Autodesk Inventor part; units mm, degrees
ref_plane "YZ Plane" through (0, 0, 0) normal (1, 0, 0) x (0, 1, 0)
ref_plane "XZ Plane" through (0, 0, 0) normal (0, 1, 0) x (-1, 0, 0)
ref_plane "XY Plane" through (0, 0, 0) normal (0, 0, 1) x (1, 0, 0)
sketch "Sketch1" plane through (0, 0, 0) normal (0, 0, 1) x (1, 0, 0)
  line L0 (0, 0) -> (20, 0)
  line L1 (20, 0) -> (20, -10)
  line L2 (20, -10) -> (0, -10)
  line L3 (0, -10) -> (0, 0)
  dimension "d0" = 20
  dimension "d1" = 10
extrude "Extrusion1" add sketch "Sketch1" along normal blind 6
sketch "Sketch2" plane through (0, 0, 0) normal (0, 1, 0) x (1, 0, 0)
  line L0 (20, 0) -> (20, -6)
  line L1 (20, 0) -> (10, 0)
  line L2 (10, 0) -> (10, -6)
  line L3 (10, -6) -> (20, -6)
  line L4 (20, -6) -> (20, 0)
  point P0 (0, 0)
  dimension "d4" = 10
extrude "Extrusion2" add sketch "Sketch2" along normal blind 1
chamfer "Chamfer2" distance 1 angle 45 1 edges at (10, 1, 3)
sketch "Sketch3" plane through (0, -10, 0) normal (0, -1, 0) x (1, 0, 0)
  line L0 (0, 6) -> (3, 6) construction
  line L1 (3, 6) -> (3, 0) construction
  line L2 (3, 0) -> (0, 0) construction
  line L3 (0, 0) -> (0, 6) construction
  line L4 (3, 6) -> (7, 6)
  line L5 (7, 6) -> (7, 0)
  line L6 (7, 0) -> (3, 0)
  line L7 (3, 0) -> (3, 6)
  line L8 (7, 6) -> (13, 6) construction
  line L9 (13, 6) -> (13, 0) construction
  line L10 (13, 0) -> (7, 0) construction
  line L11 (7, 0) -> (7, 6) construction
  line L12 (13, 6) -> (17, 6)
  line L13 (17, 6) -> (17, 0)
  line L14 (17, 0) -> (13, 0)
  line L15 (13, 0) -> (13, 6)
  dimension "d13" = 3
  dimension "d14" = 4
  dimension "d15" = 6
  dimension "d16" = 4
extrude "Extrusion3" add sketch "Sketch3" along normal blind 1
chamfer "Chamfer3" distance 1 angle 45 4 edges at (3, -11, 3) (7, -11, 3) (13, -11, 3) (17, -11, 3)
sketch "Sketch4" plane through (0, -10, 0) normal (0, -1, 0) x (1, 0, 0)
  line L0 (0, 6) -> (2.9323, 6) construction
  line L1 (0, 5) -> (2.9323, 5) construction
  line L2 (0, 0) -> (2.9323, 0) construction
  line L3 (2.9323, 1) -> (1, 1) construction
  line L4 (1, 1) -> (1, 5) construction
  line L5 (1, 5) -> (2.9323, 5) construction
  line L6 (2, 5) -> (2, 1) construction
  line L7 (1, 5) -> (2, 5)
  line L8 (2, 5) -> (2, 1)
  line L9 (2, 1) -> (1, 1)
  line L10 (1, 1) -> (1, 5)
  dimension "d22" = 1
  dimension "d23" = 1
  dimension "d24" = 1
extrude "Extrusion4" cut sketch "Sketch4" against normal blind 1
sketch "Sketch5" plane through (7, -10, 0) normal (0, -1, 0) x (1, 0, 0)
  line L0 (0, 0.2008) -> (0, 5.4827) construction
  line L1 (3, 0.2008) -> (3, 5.4827) construction
  line L2 (4, 0.2008) -> (4, 5.4827) construction
  line L3 (6, 0) -> (0.2208, 0) construction
  line L4 (6, 1) -> (0.2208, 1) construction
  line L5 (6, 6) -> (0.5976, 6) construction
  line L6 (6, 5) -> (0.5976, 5) construction
  line L7 (4, 1) -> (3, 1)
  line L8 (3, 1) -> (3, 5)
  line L9 (3, 5) -> (4, 5)
  line L10 (4, 5) -> (4, 1)
  point P0 (-7, 0)
  dimension "d27" = 3
  dimension "d28" = 1
  dimension "d29" = 1
  dimension "d30" = 1
extrude "Extrusion5" cut sketch "Sketch5" against normal blind 1
sketch "Sketch6" plane through (20, -10, 0) normal (0, -1, 0) x (1, 0, 0)
  line L0 (0, 0) -> (0, 5.7185) construction
  line L1 (-1, 0) -> (-1, 5.7185) construction
  line L2 (-2, 0) -> (-2, 5.7185) construction
  line L3 (-0.3844, 0) -> (-2.7356, 0) construction
  line L4 (-0.3844, 1) -> (-2.7356, 1) construction
  line L5 (-0.4485, 6) -> (-2.495, 6) construction
  line L6 (-0.4485, 5) -> (-2.495, 5) construction
  line L7 (-1, 1) -> (-2, 1)
  line L8 (-2, 1) -> (-2, 5)
  line L9 (-2, 5) -> (-1, 5)
  line L10 (-1, 5) -> (-1, 1)
  point P0 (-20, 0)
  dimension "d33" = 1
  dimension "d34" = 1
  dimension "d35" = 1
  dimension "d36" = 1
extrude "Extrusion6" cut sketch "Sketch6" against normal blind 1
sketch "Sketch7" plane through (0, 1, 0) normal (0, 1, 0) x (1, 0, 0)
  line L0 (11, -5.3093) -> (11, -0.576) construction
  line L1 (12.5, -5.3093) -> (12.5, -0.576) construction
  line L2 (14.5, -5.3093) -> (14.5, -0.576) construction
  line L3 (15, 0) -> (12.0712, 0) construction
  line L4 (15, -2) -> (12.0712, -2) construction
  line L5 (15, -4) -> (12.0712, -4) construction
  line L6 (14.5, -4) -> (12.5, -4)
  line L7 (12.5, -4) -> (12.5, -2)
  line L8 (12.5, -2) -> (14.5, -2)
  line L9 (14.5, -2) -> (14.5, -4)
  point P0 (0, 0)
  dimension "d39" = 1.5
  dimension "d40" = 2
  dimension "d41" = 2
  dimension "d42" = 2
extrude "Extrusion7" add sketch "Sketch7" along normal blind 1.5
sketch "Sketch8" plane through (0, 1, 0) normal (0, 1, 0) x (1, 0, 0)
  line L0 (14.5, -5.3842) -> (14.5, -1) construction
  line L1 (17.5, -5.3842) -> (17.5, -1) construction
  line L2 (18.8144, -6) -> (15.3684, -6) construction
  line L3 (18.8144, -5) -> (14.5, -5) construction
  line L4 (18.8144, -1) -> (14.5, -1) construction
  line L5 (17.5, -5) -> (18.5, -5)
  line L6 (18.5, -5) -> (18.5, -1)
  line L7 (18.5, -1) -> (17.5, -1)
  line L8 (17.5, -1) -> (17.5, -5)
  point P0 (0, 0)
  dimension "d45" = 3
  dimension "d47" = 1
  dimension "d48" = 4
  dimension "d49" = 1
extrude "Extrusion8" cut sketch "Sketch8" against normal blind 1
sketch "Sketch9" plane through (0, 0, 0) normal (0, 0, -1) x (-1, 0, 0)
  line L0 (-20, -10) -> (-0.9385, -10) construction
  line L1 (-20, -6.5) -> (-0.9385, -6.5) construction
  line L2 (-13, -10) -> (-14, -11) construction
  line L3 (-13, -10) -> (-13, -3.6474) construction
  line L4 (-3, -10) -> (-3, -3.6474) construction
  line L5 (-5, -10) -> (-5, -3.6474) construction
  line L6 (-15, -10) -> (-15, -3.6474) construction
  circle A0 centre (-15, -6.5) radius 1.5
  circle A1 centre (-5, -6.5) radius 1.5
  point P0 (0, 0)
  dimension "d52" = 3.5
  dimension "d53" = 2
  dimension "d54" = 2
  dimension "d55" = 3
  dimension "d56" = 3
extrude "Extrusion9" cut sketch "Sketch9" against normal blind 20
properties part number "Limit switch body"
Can you work these out from the model? Positions are in its coordinate system, mm. A direction names the side the tool comes from. Coordinates: 2 decimals unless noted, no trailing zeros. Order: outer loops, then holes, each group sorted by start corner. A loop starts at its lowest first (then second) coordinate and runs counter-clockwise, first axis right, second up. Notation, with made-up numbers: (2, -10) -> (59, -10) arc R10 cw to (59, -3) -> close; hole circle Ø11 at (23, 76.5). An arc over 180 degrees is marked (long way). Use one line per item in the form item = value.
Q1. Imagine slicing it at A-A, the plane z = 0.65. Give the number of separate pieces and of enclosed holes in the cut face, then the cut area to 3 significant figures.
From the geometry:
separate_pieces = 1
enclosed_holes = 2
area = 201 mm²
Q2. I need wall thicknesses on L1, parallel to Y at x = 5, z = 4.6; L2, parallel to Y at x = 15, z = 1.7; L3, parallel to X at y = -5.5, z = 2.95. Which ranges of each line are inside material? Lowest first, please.
From the geometry:
L1 = -11 to -8, -5 to 0
L2 = -11 to -8, -5 to 1
L3 = 0 to 3.88, 6.12 to 13.88, 16.12 to 20
Q3. We'd pull the mould along Z, two halves only. Please class faces 1 (the face through (10.5, 0.5, 3)), 2 (the face through (10.5, -9.5, 5)), 3 (the face through (14, 2, 4)): released by +Z, released by -Z, zero draft, split by the parting line, or undercut.
From the geometry:
face_1 = zero draft
face_2 = undercut
face_3 = released by +Z
Q4. Will these pins go through, and if not, where does the flat tip stop? P1, Ø3, axis at x = 17.5, z = 3, coming from the +Y side; P2, Ø0.8, axis at x = 1.5, z = 4, coming from the -Y side; P3, Ø0.8, axis at y = 0.5, z = 2, coming from the -X side.
From the geometry:
P1 = 1
P2 = -9
P3 = 10.1
Q5. Imagine slicing it at B-B, the plane x = 5. List the corners of the cut face in (y, z) for me.
From the geometry:
outline = (-11, 0) -> (-8, 0) -> (-8, 6) -> (-11, 6) -> close; (-5, 0) -> (0, 0) -> (0, 6) -> (-5, 6) -> close
Q6. Imagine slicing it at D-D, the plane x = 15. List the corners of the cut face in (y, z) for me, then the cut area to 3 significant figures.
From the geometry:
outline = (-11, 0) -> (-8, 0) -> (-8, 6) -> (-11, 6) -> close; (-5, 0) -> (1, 0) -> (1, 6) -> (-5, 6) -> close
area = 54.0 mm²
Q7. Which directions (+Z, -Z, +X, -X, +Y, -Y) give clear straight access to the entire face, cutting with the end or side of a thin tool? Please do faces 4 (the face through (12.5, 2, 3)), 5 (the face through (18, 0, 3)), 6 (the face through (11, -9.5, 3)), 7 (the face through (13, 2, 2)).
From the geometry:
face_4 = +Z, -Z, -X, +Y
face_5 = +Y
face_6 = -Y
face_7 = -Z, +X, -X, +Y
Q8. Imagine slicing it at C-C, the plane y = -6.5. List the corners of the cut face in (x, z) for me, then the cut area to 3 significant figures.
From the geometry:
outline = (0, 0) -> (3.5, 0) -> (3.5, 6) -> (0, 6) -> close; (6.5, 0) -> (13.5, 0) -> (13.5, 6) -> (6.5, 6) -> close; (16.5, 0) -> (20, 0) -> (20, 6) -> (16.5, 6) -> close
area = 84.0 mm²
